Could you check a few things on this model? Use its own coordinates, in mm. Face numbers are marked on the shaded views. A direction names the side the tool comes from. Coordinates: 2 decimals unless noted, no trailing zeros. Order: outer loops, then holes, each group sorted by start corner. A loop starts at its lowest first (then second) coordinate and runs counter-clockwise, first axis right, second up. Notation, with made-up numbers: (-26, 42) - (-7, 42) arc R29 cw to (-7, 65) - close; hole circle Ø10 at (70, -37.5). An arc over 180 degrees is marked (long way). One line per item, written item: value. Start each with the question number.
from build123d import *

# Parameters (mm, degrees)
SKETCH001_R        = 4.5
SKETCH001_R_2      = 2.5
PAD001_DEPTH       = 9
SKETCH_W           = 8
SKETCH_H           = 7
POCKET_DEPTH       = 4.5
SKETCH006_R        = 5
PAD_DEPTH          = 4
SKETCH004_W        = 4.5
SKETCH004_H        = 3.4
POCKET001_DEPTH    = 5
POLARPATTERN_COUNT = 2
SKETCH007_R        = 1.7
POCKET002_DEPTH    = 4
FILLET_R           = 1
CHAMFER_SIZE       = 2
FILLET001_R        = 0.9


with BuildPart() as part:
    # Sketch001 → Pad001 (new body, symmetric)
    with BuildSketch(Plane.YZ):
        with Locations((0, 4.5)):
            Circle(SKETCH001_R)
        with Locations((0, 4.5)):
            Circle(SKETCH001_R_2, mode=Mode.SUBTRACT)
    extrude(amount=PAD001_DEPTH, both=True)

    # Sketch → Pocket (cut, symmetric)
    with BuildSketch(Plane.XZ):
        with Locations((0, 5.5)):
            Rectangle(SKETCH_W, SKETCH_H)
    extrude(amount=POCKET_DEPTH, both=True, mode=Mode.SUBTRACT)

    # Sketch006 → Pad (join)
    with BuildSketch(Plane(origin=(0, 0, 2), x_dir=(0, -1, 0), z_dir=(0, 0, 1))):
        Circle(SKETCH006_R)
    extrude(amount=-PAD_DEPTH)

    # Sketch004 → Pocket001 (cut)
    with BuildSketch(Plane.YZ.offset(9)):
        with Locations((2.25, 3.7)):
            Rectangle(SKETCH004_W, SKETCH004_H)
    pocket001 = extrude(amount=-POCKET001_DEPTH, mode=Mode.SUBTRACT)

    # PolarPattern: Pocket001 ×2 about axis
    polarpattern_axis = Axis((0, 0, 0), (0, 0, 1))
    for i in range(1, POLARPATTERN_COUNT):
        add(pocket001.rotate(polarpattern_axis, i * 360 / POLARPATTERN_COUNT), mode=Mode.SUBTRACT)

    # Sketch007 (on Face9 of Pad) → Pocket002 (cut)
    with BuildSketch(Plane(origin=(0, 0, 2), x_dir=(0, -1, 0), z_dir=(0, 0, 1))):
        Circle(SKETCH007_R)
    extrude(amount=-POCKET002_DEPTH, mode=Mode.SUBTRACT)

    # Fillet
    fillet_edges = [part.edges().sort_by_distance(p)[0] for p in [
        (-5, 0, 0),
        (5, 0, 0),
    ]]
    fillet(fillet_edges, radius=FILLET_R)

    # Chamfer
    chamfer_edges = [part.edges().sort_by_distance(p)[0] for p in [
        (1.202082, -1.202082, 2),
    ]]
    chamfer(chamfer_edges, length=CHAMFER_SIZE)

    # Fillet001
    fillet001_edges = [part.edges().sort_by_distance(p)[0] for p in [
        (6.5, 2.332381, 5.4),
        (6.5, 4.409082, 5.4),
        (-6.5, -2.332381, 5.4),
        (-6.5, -4.409082, 5.4),
    ]]
    fillet(fillet001_edges, radius=FILLET001_R)


solid = part.part
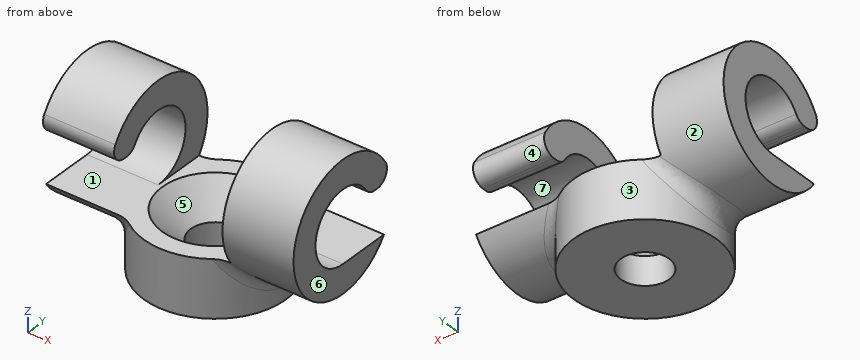
Q1. We'd pull the mould along Y, two halves only. Please class the marked faces 4, 5, 6 and 7: +Y half, -Y half, draft (parallel to the pull), parting line (faces both ways), or undercut.
Q2. If I drill on L1, parallel to X at y = 0.5, z = 8.25; L2, parallel to Z at x = 7.7, y = 0; L3, parallel to X at y = 0, z = -1.25, over which ranges is the centre line in solid material (lowest first)?
Q3. Which directions (+Z, -Z, +X, -X, +Y, -Y) give clear straight access to the entire face, cutting with the end or side of a thin tool? Please do the marked faces 1, 2 and 3.
Q4. I want a section at C-C on y = -1.5. State how many separate pieces and enclosed holes the cut face has, then the cut area to 3 significant figures.
Q5. I want a section at A-A on x = 0. Please give me the cut outline in (y, z).
Q6. I want a section at B-B on z = 4.5. Please give me the cut outline in (x, y).
Q7. I'm going to push flat-ended pins straight in: pin 1 (4.5 mm diameter, centred on y = 0, z = 4.5, fed in from -X); pin 2 (5.5 mm diameter, centred on x = 0, y = 0, fed in from +Z); pin 3 (5 mm diameter, centred on x = 2.5, y = -2.5, fed in from +Z); pin 4 (5 mm diameter, centred on x = 0.5, y = 2.5, fed in from +Z). Where does each tip first touch, or does it pass through?
Q8. I want a section at D-D on z = 3. Please give me the cut outline in (x, y), then the cut area to 3 significant figures.
Values follow:
1. face 4: +Y half
1. face 5: undercut
1. face 6: draft
1. face 7: undercut
2. L1: x = -9 to -4, 4 to 9
2. L2: z = 0 to 2, 7 to 9
2. L3: x = -5 to -1.7, 1.7 to 5
3. face 1: none
3. face 2: -X
3. face 3: -Z
4. separate pieces: 4
4. enclosed holes: 0
4. area: 66.2 mm^2
5. outline: (-5, -2) - (-1.7, -2) - (-1.7, 0) - (-3.7, 2) - (-5, 2) - close; (1.7, -2) - (5, -2) - (5, 2) - (3.7, 2) - (1.7, 0) - close
6. outline: (-9, 2.5) - (-4, 2.5) - (-4, 4.5) - (-9, 4.5) - close; (4, -4.5) - (9, -4.5) - (9, -2.5) - (4, -2.5) - close
7. pin 1: passes through
7. pin 2: stops at z = 1.05
7. pin 3: stops at z = 8.97
7. pin 4: stops at z = 2
8. outline: (-9, 2) - (-4, 2) - (-4, 4.24) - (-9, 4.24) - close; (4, -4.24) - (9, -4.24) - (9, -2) - (4, -2) - close
8. area: 22.4 mm^2
